Build history of the part. All positions in model axes, mm. A direction names the side the tool comes from. Give positions to 0.01 mm unless a question says otherwise; leave off trailing zeros. Order: outer loops, then holes, each group sorted by start corner. A loop starts at its lowest first (then second) coordinate and runs counter-clockwise, first axis right, second up. Notation, with made-up numbers: (-8, 59) - (18, 59) arc R15 ccw to (18, 74) - close; hole circle Ø8 at (-3, -9). An arc over 180 degrees is marked (long way). Use a Markdown table: item, result. Add a question column.
(1) Flat gauge pins, fed straight in: pin 1 (2.5 mm diameter, centred on y = -46, z = 241.5, fed in from -X); pin 2 (5 mm diameter, centred on y = -25, z = 230.5, fed in from -X); pin 3 (3.5 mm diameter, centred on y = 96.5, z = 247, fed in from +X). Where does each tip first touch, or does it go through?
(2) Slice it at C-C (y = 0). Write the cut outline in (x, z), then the cut area to 3 significant figures.
(3) Which spindle directions (+Z, -Z, +X, -X, +Y, -Y) get a long thin tool onto all of the face, cutting with end or side? Do faces 5 (the face through (-68, -48, 237)), 6 (the face through (-90, 93, 244)), 7 (the face through (-85, 98, 243)). Say none if no direction does.
(4) Wall check: line 1 (Y direction, x = -46, z = 246.2); line 2 (Y direction, x = -49.5, z = 223); line 3 (X direction, y = 98, z = 246.15). Give the ranges that are in metal, low to high.
(5) Slice it at D-D (x = -67.5). Write the cut outline in (y, z), then the cut area to 3 significant figures.
(6) Slice it at B-B (x = -55). Write the cut outline in (y, z), then the cut area to 3 significant figures.
(7) Slice it at A-A (y = 98). Write the cut outline in (x, z), then the cut area to 3 significant figures.
(8) Mould opens along X. For faces 1 (the face through (-79.5, 66.8, 243.6)), 2 (the face through (-69, -50, 241)), 3 (the face through (-63, 22, 248)), 4 (the face through (-47.474, 1.352, 246.479)) say: +X half, -X half, draft (parallel to the pull), parting line (faces both ways), or undercut.
from build123d import *

# Parameters (mm, degrees)
SKETCH250_W       = 8
SKETCH250_H       = 8
SKETCH250_R       = 1.75
PAD023_DEPTH      = 3
SKETCH252_W       = 44
SKETCH252_H       = 150
SKETCH252_R       = 2
PAD024_DEPTH      = 3
PAD025_DEPTH      = 59
PAD026_DEPTH      = 30
SKETCH255_W       = 16
SKETCH255_H       = 13
PAD027_DEPTH      = 3
SKETCH256_R       = 1.85
PAD028_DEPTH      = 3
PAD028_DEPTH_BACK = 5
SKETCH257_W       = 32
SKETCH257_H       = 19
POCKET018_DEPTH   = 5


with BuildPart() as part:
    # Sketch250 → Pad023 (new body)
    with BuildSketch(Plane.YZ):
        Rectangle(SKETCH250_W, SKETCH250_H)
        Circle(SKETCH250_R, mode=Mode.SUBTRACT)
    extrude(amount=PAD023_DEPTH)

    # Sketch252 → Pad024 (join)
    with BuildSketch(Plane.XY.offset(4)):
        with Locations((6, 63)):
            Rectangle(SKETCH252_W, SKETCH252_H)
        with Locations((5, 48)):
            Circle(SKETCH252_R, mode=Mode.SUBTRACT)
        with Locations((14, 48)):
            Circle(SKETCH252_R, mode=Mode.SUBTRACT)
        with Locations((23, 48)):
            Circle(SKETCH252_R, mode=Mode.SUBTRACT)
        with Locations((23, 124.6)):
            Circle(SKETCH252_R, mode=Mode.SUBTRACT)
        with Locations((14, 124.6)):
            Circle(SKETCH252_R, mode=Mode.SUBTRACT)
        with Locations((5, 124.6)):
            Circle(SKETCH252_R, mode=Mode.SUBTRACT)
    extrude(amount=PAD024_DEPTH)

    # Sketch253 → Pad025 (join)
    with BuildSketch(Plane.XY.offset(7)):
        Polygon((0, 139.9), (0, 138), (28, 138), (28, -12), (0, -12), (0, -13.9), (30, -13.9), (30, 139.9), align=None)
    extrude(amount=-PAD025_DEPTH)

    # Sketch254 → Pad026 (join)
    with BuildSketch(Plane.XZ.offset(-100)):
        with BuildLine():
            ThreePointArc((-6, 4), (-4.6, 2.6), (-3.2, 4))
            Line((-6, 4), (-3.2, 4))
        make_face()
        with BuildLine():
            ThreePointArc((-11.9, 4), (-10.5, 2.6), (-9.1, 4))
            Line((-11.9, 4), (-9.1, 4))
        make_face()
    extrude(amount=-PAD026_DEPTH)

    # Sketch255 → Pad027 (join)
    with BuildSketch(Plane.XY.offset(4)):
        with Locations((-8, 144.5)):
            Rectangle(SKETCH255_W, SKETCH255_H)
    extrude(amount=PAD027_DEPTH)

    # Sketch256 → Pad028 (join, two sides)
    with BuildSketch(Plane.XY.offset(4)) as pad028_sk:
        with BuildLine():
            Line((-16, 141), (-27, 141))
            ThreePointArc((-27, 151), (-32, 146), (-27, 141))
            Line((-27, 151), (-16, 151))
            Line((-16, 151), (-16, 141))
        make_face()
        with Locations((-27, 146)):
            Circle(SKETCH256_R, mode=Mode.SUBTRACT)
    extrude(amount=PAD028_DEPTH)
    extrude(pad028_sk.sketch, amount=-PAD028_DEPTH_BACK)

    # Sketch257 → Pocket018 (cut)
    with BuildSketch(Plane.XZ.offset(14)):
        with Locations((12, -43.5)):
            Rectangle(SKETCH257_W, SKETCH257_H)
    extrude(amount=-POCKET018_DEPTH, mode=Mode.SUBTRACT)


with BuildPart() as part_1:
    # Body012 placement: moved
    add(part.part.moved(Location((-69, -48, 241))))


solid = part_1.part
Solution:
| question | item | result |
|---|---|---|
| 1 | pin 1 | x = -69 |
| 1 | pin 2 | x = -41 |
| 1 | pin 3 | x = -69 |
| 2 | outline | (-85, 245) - (-66, 245) - (-66, 248) - (-85, 248) - close; (-62, 245) - (-57, 245) - (-57, 248) - (-62, 248) - close; (-53, 245) - (-48, 245) - (-48, 248) - (-53, 248) - close; (-44, 245) - (-41, 245) - (-41, 189) - (-39, 189) - (-39, 248) - (-44, 248) - close |
| 2 | area | 214 mm2 |
| 3 | face 5 | -Z, -X |
| 3 | face 6 | +Z, -Z, -X, -Y |
| 3 | face 7 | -Z, +X, +Y, -Y |
| 4 | line 1 | -61.9 to -2, 2 to 74.6, 78.6 to 91.9 |
| 4 | line 2 | -61.9 to -60, 90 to 91.9 |
| 4 | line 3 | -101 to -97.85, -94.15 to -69 |
| 5 | outline | (-61.9, 207) - (-60, 207) - (-60, 245) - (-52, 245) - (-52, 237) - (-44, 237) - (-44, 245) - (90, 245) - (90, 189) - (91.9, 189) - (91.9, 248) - (-61.9, 248) - close; hole circle Ø3.5 at (-48, 241) |
| 5 | area | 694 mm2 |
| 6 | outline | (-61.9, 207) - (-60, 207) - (-60, 245) - (-2, 245) - (-2, 248) - (-61.9, 248) - close; (2, 245) - (74.6, 245) - (74.6, 248) - (2, 248) - close; (78.6, 245) - (90, 245) - (90, 189) - (91.9, 189) - (91.9, 248) - (78.6, 248) - close |
| 6 | area | 616 mm2 |
| 7 | outline | (-101, 240) - (-97.85, 240) - (-97.85, 248) - (-101, 248) - close; (-94.15, 240) - (-85, 240) - (-85, 245) - (-69, 245) - (-69, 248) - (-94.15, 248) - close |
| 7 | area | 146 mm2 |
| 8 | face 1 | undercut |
| 8 | face 2 | -X half |
| 8 | face 3 | draft |
| 8 | face 4 | undercut |
